Here's how the part is built. I have some questions about the finished solid (model axes, mm). Coordinates: 2 decimals unless noted, no trailing zeros. Write each loop counter-clockwise with the first axis right and the second up, starting at its lowest first coordinate (ties: lowest second). Pieces come first, ordered by that corner, then holes. Notation, with made-up numbers: M -18,85 L 29,85 A34 ccw 29,121 Z; hole C 70.5,28 d5. An arc over 180 degrees is marked long. Use a Markdown table: item, result.
Autodesk Inventor part; units mm, degrees
ref_plane "YZ Plane" through (0, 0, 0) normal (1, 0, 0) x (0, 1, 0)
ref_plane "XZ Plane" through (0, 0, 0) normal (0, 1, 0) x (-1, 0, 0)
ref_plane "XY Plane" through (0, 0, 0) normal (0, 0, 1) x (1, 0, 0)
sketch "Esboço1" plane through (0, 0, 0) normal (0, 1, 0) x (-1, 0, 0)
  circle A0 centre (0, 0) radius 34.95
  circle A1 centre (0, 0) radius 1.5
  line L0 (36, 66.1815) -> (-36, 66.1815)
  line L1 (-36, 66.1815) -> (-36, -66.1815)
  line L2 (-36, -66.1815) -> (36, -66.1815)
  line L3 (36, -66.1815) -> (36, 66.1815)
  line L4 (36, 66.1815) -> (-36, -66.1815) construction
  line L5 (-36, 66.1815) -> (36, -66.1815) construction
  dimension "d0" = 69.9
  dimension "d3" = 3
  dimension "d11" = 132.363
  dimension "d12" = 72
extrude "Extrusão1" add sketch "Esboço1" along normal blind 12 contours A0 | L3 L2 L1 L0
sketch "Esboço2" plane through (0, 0, 0) normal (0, -1, 0) x (1, 0, 0)
  circle A0 centre (0, 0) radius 1.5
  circle A1 centre (0, 0) radius 26
  circle A2 centre (0, -26) radius 2.1
  circle A3 centre (0, 26) radius 2.1
  circle A4 centre (0, 53.1) radius 5
  circle A5 centre (0, -53.1) radius 5
  dimension "d4" = 4.2
  dimension "d5" = 4.2
  dimension "d13" = 10
  dimension "d14" = 53.1
  dimension "d15" = 10
  dimension "d16" = 53.1
  dimension "d20" = 52
extrude "Extrusão2" cut sketch "Esboço2" against normal blind 12 contours A3 A1 | A1 A3 | A2 A1 | A1 A2 | A4 | A5
chamfer "Chanfro1" distance 2.5 angle 45 2 edges at (-2.1, 0, 26) (-2.1, 0, -26)
fillet "Arredondamento1" radius 10 4 edges at (-36, 6, -66.1815) (36, 6, -66.1815) (36, 6, 66.1815) (-36, 6, 66.1815)
sketch "Esboço3" plane through (0, 0, 0) normal (0, -1, 0) x (1, 0, 0)
  circle A0 centre (28, -28) radius 4
  circle A1 centre (0, 0) radius 1.5
  line L0 (0, 0) -> (13.6078, 0)
  line L1 (13.6078, 0) -> (13.6078, -9.8158)
  line L2 (13.6078, -9.8158) -> (0, -9.8158)
  line L3 (0, -9.8158) -> (0, 0)
  circle A2 centre (28, 28) radius 4
  circle A3 centre (-28, -28) radius 4
  circle A4 centre (-28, 28) radius 4
  dimension "d22" = 8
  dimension "d23" = 28
  dimension "d24" = 28
  dimension "d27" = 56
  dimension "d30" = 56
extrude "Extrusão3" cut sketch "Esboço3" against normal blind 12 contours A0 | A2 | A3 | A4
properties part number "Inferior_base"
1. Suppose I cut it at D-D on z = -26. Write out the boundary of the cut face in (x, y).
Answers follow:
| item | result |
|---|---|
| outline | M -36,0 L -31.46,0 L -31.46,12 L -36,12 Z; M -24.54,0 L -4.6,0 L -2.1,2.5 L -2.1,12 L -24.54,12 Z; M 2.1,2.5 L 4.6,0 L 24.54,0 L 24.54,12 L 2.1,12 Z; M 31.46,0 L 36,0 L 36,12 L 31.46,12 Z |
2. I need wall thicknesses on probe 1 along Z at (x, y) = (0, 6.25); probe 2 along X at (y, z) = (6, 26); probe 3 along Z at (x, y) = (-26.5, 10). Which ranges of each line are inside material? Lowest first, please.
Answers follow:
| item | result |
|---|---|
| probe 1 | z = -66.18 to -58.1, -48.1 to -28.1, -23.9 to -1.5, 1.5 to 23.9, 28.1 to 48.1, 58.1 to 66.18 |
| probe 2 | x = -36 to -31.46, -24.54 to -2.1, 2.1 to 24.54, 31.46 to 36 |
| probe 3 | z = -66.17 to -31.71, -24.29 to 24.29, 31.71 to 66.17 |
3. We'd pull the mould along Z, two halves only. Please class faces 1 (the face through (-28.521, 5.916, 31.966)), 2 (the face through (-36, 6, -1)), 3 (the face through (-1.08, 5.92, 48.22)), 4 (the face through (0, 6, 66.182)): +Z half, -Z half, draft (parallel to the pull), parting line (faces both ways), or undercut.
Answers follow:
| item | result |
|---|---|
| face 1 | undercut |
| face 2 | draft |
| face 3 | undercut |
| face 4 | +Z half |
4. Suppose I cut it at B-B on y = 10.25. State how many separate pieces and enclosed holes the cut face has, and give its area (3 significant figures).
Answers follow:
| item | result |
|---|---|
| separate pieces | 1 |
| enclosed holes | 9 |
| area | 9,050 mm2 |
5. Will this pin go through, and if not, where does the flat tip stop? pin 1 Ø5 at (x, z) = (-28, -28) entering from +Y.
Answers follow:
| item | result |
|---|---|
| pin 1 | passes through |
6. Suppose I cut it at C-C on x = 0. Write out the boundary of the cut face in (y, z).
Answers follow:
| item | result |
|---|---|
| outline | M 0,-66.18 L 12,-66.18 L 12,-58.1 L 0,-58.1 Z; M 0,-48.1 L 12,-48.1 L 12,-28.1 L 2.5,-28.1 L 0,-30.6 Z; M 0,-21.4 L 2.5,-23.9 L 12,-23.9 L 12,-1.5 L 0,-1.5 Z; M 0,1.5 L 12,1.5 L 12,23.9 L 2.5,23.9 L 0,21.4 Z; M 0,30.6 L 2.5,28.1 L 12,28.1 L 12,48.1 L 0,48.1 Z; M 0,58.1 L 12,58.1 L 12,66.18 L 0,66.18 Z |
7. Suppose I cut it at A-A on z = 53.1. Write out the boundary of the cut face in (x, y).
Answers follow:
| item | result |
|---|---|
| outline | M -36,0 L -5,0 L -5,12 L -36,12 Z; M 5,0 L 36,0 L 36,12 L 5,12 Z |
